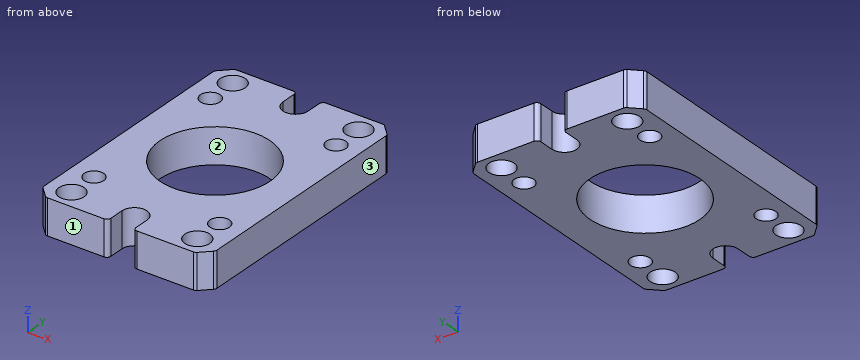
```python
from build123d import *

# Parameters (mm, degrees)
ESBO_O1_R                = 7
ESBO_O1_R_2              = 1.6
ESBO_O1_R_3              = 1.25
RESSALTO_EXTRUS_O1_DEPTH = 4.5


with BuildPart() as part:
    # Esboço1 → Ressalto-extrusão1 (new body)
    with BuildSketch(Plane(origin=(0, 0, 0), x_dir=(-1, 0, 0), z_dir=(0, 0, -1))):
        with BuildLine():
            Line((-2.1, 16.25), (-9.292893219, 16.25))
            ThreePointArc((-9.292893219, 16.25), (-9.484234935, 16.211939766), (-9.646446609, 16.103553391))
            Line((-9.646446609, 16.103553391), (-10.853553391, 14.896446609))
            ThreePointArc((-10.853553391, 14.896446609), (-10.961939766, 14.734234935), (-11, 14.542893219))
            Line((-11, 14.542893219), (-11, -14.542893219))
            ThreePointArc((-11, -14.542893219), (-10.961939766, -14.734234935), (-10.853553391, -14.896446609))
            Line((-10.853553391, -14.896446609), (-9.646446609, -16.103553391))
            ThreePointArc((-9.646446609, -16.103553391), (-9.484234935, -16.211939766), (-9.292893219, -16.25))
            Line((-9.292893219, -16.25), (-2.1, -16.25))
            ThreePointArc((-2.1, -16.25), (-1.746446609, -16.103553391), (-1.6, -15.75))
            Line((-1.6, -15.75), (-1.6, -13.856406461))
            ThreePointArc((-1.6, -13.856406461), (0, -12.256406461), (1.6, -13.856406461))
            Line((1.6, -13.856406461), (1.6, -15.75))
            ThreePointArc((1.6, -15.75), (1.746446609, -16.103553391), (2.1, -16.25))
            Line((2.1, -16.25), (9.292893219, -16.25))
            ThreePointArc((9.292893219, -16.25), (9.484234935, -16.211939766), (9.646446609, -16.103553391))
            Line((9.646446609, -16.103553391), (10.853553391, -14.896446609))
            ThreePointArc((10.853553391, -14.896446609), (10.961939766, -14.734234935), (11, -14.542893219))
            Line((11, -14.542893219), (11, 14.542893219))
            ThreePointArc((11, 14.542893219), (10.961939766, 14.734234935), (10.853553391, 14.896446609))
            Line((10.853553391, 14.896446609), (9.646446609, 16.103553391))
            ThreePointArc((9.646446609, 16.103553391), (9.484234935, 16.211939766), (9.292893219, 16.25))
            Line((9.292893219, 16.25), (2.1, 16.25))
            ThreePointArc((2.1, 16.25), (1.746446609, 16.103553391), (1.6, 15.75))
            Line((1.6, 15.75), (1.6, 13.856406461))
            ThreePointArc((1.6, 13.856406461), (0, 12.256406461), (-1.6, 13.856406461))
            Line((-1.6, 13.856406461), (-1.6, 15.75))
            ThreePointArc((-1.6, 15.75), (-1.746446609, 16.103553391), (-2.1, 16.25))
        make_face()
        Circle(ESBO_O1_R, mode=Mode.SUBTRACT)
        with Locations((-8, -13.85640646)):
            Circle(ESBO_O1_R_2, mode=Mode.SUBTRACT)
        with Locations((8, -13.85640646)):
            Circle(ESBO_O1_R_2, mode=Mode.SUBTRACT)
        with Locations((8, 13.85640646)):
            Circle(ESBO_O1_R_2, mode=Mode.SUBTRACT)
        with Locations((-8, 13.85640646)):
            Circle(ESBO_O1_R_2, mode=Mode.SUBTRACT)
        with Locations((-8, -10)):
            Circle(ESBO_O1_R_3, mode=Mode.SUBTRACT)
        with Locations((8, -10)):
            Circle(ESBO_O1_R_3, mode=Mode.SUBTRACT)
        with Locations((8, 10)):
            Circle(ESBO_O1_R_3, mode=Mode.SUBTRACT)
        with Locations((-8, 10)):
            Circle(ESBO_O1_R_3, mode=Mode.SUBTRACT)
    extrude(amount=-RESSALTO_EXTRUS_O1_DEPTH)


solid = part.part
```
The listing builds one solid part. Answer for the finished solid, in the listing's coordinates (mm). Face numbers are marked on the shaded views. Give positions to 0.01 mm unless a question says otherwise; leave off trailing zeros. Order: outer loops, then holes, each group sorted by start corner. A loop starts at its lowest first (then second) coordinate and runs counter-clockwise, first axis right, second up.
Item 1: The part is cut by section D-D, the plane x = -3. Give the vertices of the cut face in (y, z).
From the geometry:
outline: (-16.25, 0) - (-6.32, 0) - (-6.32, 4.5) - (-16.25, 4.5) - close; (6.32, 0) - (16.25, 0) - (16.25, 4.5) - (6.32, 4.5) - close
Item 2: The part is cut by section C-C, the plane y = -3. Give the vertices of the cut face in (x, z).
From the geometry:
outline: (-11, 0) - (-6.32, 0) - (-6.32, 4.5) - (-11, 4.5) - close; (6.32, 0) - (11, 0) - (11, 4.5) - (6.32, 4.5) - close
Item 3: The part is cut by section A-A, the plane x = -8. Give the vertices of the cut face in (y, z), and give its area (4 significant figures).
From the geometry:
outline: (-16.25, 0) - (-15.46, 0) - (-15.46, 4.5) - (-16.25, 4.5) - close; (-12.26, 0) - (-11.25, 0) - (-11.25, 4.5) - (-12.26, 4.5) - close; (-8.75, 0) - (8.75, 0) - (8.75, 4.5) - (-8.75, 4.5) - close; (11.25, 0) - (12.26, 0) - (12.26, 4.5) - (11.25, 4.5) - close; (15.46, 0) - (16.25, 0) - (16.25, 4.5) - (15.46, 4.5) - close
area: 94.95 mm2
Item 4: The part is cut by section B-B, the plane y = 10. Give the vertices of the cut face in (x, z), and give its area (3 significant figures).
From the geometry:
outline: (-11, 0) - (-9.25, 0) - (-9.25, 4.5) - (-11, 4.5) - close; (-6.75, 0) - (6.75, 0) - (6.75, 4.5) - (-6.75, 4.5) - close; (9.25, 0) - (11, 0) - (11, 4.5) - (9.25, 4.5) - close
area: 76.5 mm2
Item 5: For a pull along X with two mould halves and no side action, classify the marked faces 1, 2 and 3 as pulls with the +X half, pulls with the -X half, needs draft (parallel to the pull), parting line crosses it, or undercut.
From the geometry:
face 1: needs draft
face 2: undercut
face 3: pulls with the +X half
Item 6: Find the intervals of material crossed by probe 1 along X at (y, z) = (-14, 2.2); probe 2 along Y at (x, z) = (-8, 2.45); probe 3 along X at (y, z) = (-5, 0.85), in increasing order.
From the geometry:
probe 1: x = -11 to -9.59, -6.41 to -1.6, 1.6 to 6.41, 9.59 to 11
probe 2: y = -16.25 to -15.46, -12.26 to -11.25, -8.75 to 8.75, 11.25 to 12.26, 15.46 to 16.25
probe 3: x = -11 to -4.9, 4.9 to 11
